from build123d import *

# Parameters (mm, degrees)
SKETCH_R     = 2.2
PAD_DEPTH    = 4
PAD001_DEPTH = 11
POCKET_DEPTH = 2
FILLET_R     = 6.46
CHAMFER_SIZE = 0.6
PAD002_DEPTH = 0.9


with BuildPart() as revolution:
    # Sketch002 → Revolution (revolve)
    with BuildSketch(Plane.XZ):
        Polygon((9.9, 11.25), (10.5, 11.85), (10.5, 7.15), (9.9, 7.75), align=None)
    revolve(axis=Axis((0, 0, 0), (0, 0, 1)))


with BuildPart() as pad002:
    # Sketch → Pad (new body)
    with BuildSketch(Plane.XY):
        with BuildLine():
            Line((-10.212408, -2.440639), (-19.784288, -2.440639))
            Line((-19.784288, -2.440639), (-19.784288, 10.5))
            Line((19.784288, 10.5), (-19.784288, 10.5))
            Line((19.784288, -2.440639), (19.784288, 10.5))
            Line((10.212408, -2.440639), (19.784288, -2.440639))
            ThreePointArc((7.424621, -7.424621), (9.163854, -5.125795), (10.212408, -2.440639))
            Line((5.674532, -5.674532), (7.424621, -7.424621))
            ThreePointArc((5.674532, -5.674532), (0, 8.025), (-5.674532, -5.674532))
            Line((-5.674532, -5.674532), (-7.424621, -7.424621))
            ThreePointArc((-10.212408, -2.440639), (-9.163854, -5.125795), (-7.424621, -7.424621))
        make_face()
        with Locations((13.859288, 4.029681)):
            Circle(SKETCH_R, mode=Mode.SUBTRACT)
        with Locations((-13.859288, 4.029681)):
            Circle(SKETCH_R, mode=Mode.SUBTRACT)
    extrude(amount=PAD_DEPTH)

    # Sketch001 → Pad001 (new body)
    with BuildSketch(Plane.XY.offset(4)):
        with BuildLine():
            ThreePointArc((5.674532, -5.674532), (0, 8.025), (-5.674532, -5.674532))
            Line((-5.674532, -5.674532), (-7.424621, -7.424621))
            ThreePointArc((7.424621, -7.424621), (0, 10.5), (-7.424621, -7.424621))
            Line((5.674532, -5.674532), (7.424621, -7.424621))
        make_face()
    extrude(amount=PAD001_DEPTH)

    # Cut: cut Revolution
    add(revolution.part, mode=Mode.SUBTRACT)

    # Sketch003 → Pocket (cut)
    with BuildSketch(Plane.XY.offset(4)):
        Polygon((17.812321, 3.059611), (16.675909, 6.968072), (12.722877, 7.938142), (9.906256, 4.99975), (11.042667, 1.091289), (14.995699, 0.121219), align=None)
        Polygon((-17.812321, 3.059611), (-14.995699, 0.121219), (-11.042667, 1.091289), (-9.906256, 4.99975), (-12.722877, 7.938142), (-16.675909, 6.968072), align=None)
    extrude(amount=-POCKET_DEPTH, mode=Mode.SUBTRACT)

    # Fillet
    fillet_edges = [pad002.edges().sort_by_distance(p)[0] for p in [
        (19.784288, -2.440639, 2),
        (19.784288, 10.5, 2),
        (-19.784288, 10.5, 2),
        (-19.784288, -2.440639, 2),
    ]]
    fillet(fillet_edges, radius=FILLET_R)

    # Chamfer
    chamfer_edges = [pad002.edges().sort_by_distance(p)[0] for p in [
        (0, 10.5, 0),
        (17.892198, 8.60791, 0),
        (-17.892198, 8.60791, 0),
    ]]
    chamfer(chamfer_edges, length=CHAMFER_SIZE)

    # Sketch004 → Pad002 (new body)
    with BuildSketch(Plane(origin=(0, 0, 0), x_dir=(1, 0, 0), z_dir=(0, 0, -1))):
        with BuildLine():
            ThreePointArc((-4.949747, 4.949747), (0, -7), (4.949747, 4.949747))
            Line((4.949747, 4.949747), (5.674532, 5.674532))
            ThreePointArc((-5.674532, 5.674532), (0, -8.025), (5.674532, 5.674532))
            Line((-5.674532, 5.674532), (-4.949747, 4.949747))
        make_face()
    extrude(amount=-PAD002_DEPTH)


solid = pad002.part
Geometry check sheet. Reference: the model listing, model coordinates, mm. A direction names the side the tool comes from. Give positions to 0.01 mm unless a question says otherwise; leave off trailing zeros. Loops run counter-clockwise (first coordinate to the right, second up) from the corner with the lowest first, then second, coordinate; pieces in that order, holes last. Notation, with made-up numbers: M 82,64.25 L 92,64.25 A30 cw 92,87.25 Z; hole C -13.75,-27 d7. An arc over 180 degrees is marked long. Answer as a JSON object with one key per item and string values. Group by question number.
Item 1: Mould release check, pull along Y, two halves, no side actions. Record for faces 1 (the flat face through (0, 9, 0)), 2 (the flat face through (0, 10.5, 2)), 3 (the flat face through (10.467, 3.073, 3.014)): pulls with the +Y half, pulls with the -Y half, needs draft (parallel to the pull), parting line crosses it, or undercut.
Item 2: Gauge pin test, flat ends, axial feed: pin 1 (2 mm diameter, centred on x = 5, z = 8.5, fed in from +Y); pin 2 (8.5 mm diameter, centred on x = 0, y = 0, fed in from +Z); pin 3 (2 mm diameter, centred on y = 7.5, z = 7.5, fed in from -X); pin 4 (2 mm diameter, centred on x = 2.5, z = 3, fed in from -Y). Record the tip position at first contact, or that the pin passes through.
Item 3: Material ranges on L1, parallel to Z at x = 12.5, y = 0.25; L2, parallel to X at y = 6.5, z = 12; L3, parallel to X at y = -3.75, z = 2, recorded low to high.
Item 4: Sectioned sample at C-C on z = 4.75. Record the boundary of the cut face in (x, y) (3 decimals).
Item 5: Sectioned sample at A-A on z = 2.5. Record the boundary of the cut face in (x, y) (3 decimals).
Item 6: Access from +Z, -Z, +X, -X, +Y, -Y to the whole of each face (thin tool, end or side, straight path). Record for faces 4 (the conical face through (0.332, 10.057, 7.588)), 5 (the flat face through (-11.295, 6.448, 3.014)), 6 (the flat face through (-12, -2.441, 2)).
Item 7: Sectioned sample at B-B on z = 8.5. Record the boundary of the cut face in (x, y) (3 decimals), plus the area to 3 significant figures.
Findings below:
{
 "1": {"face 1": "needs draft", "face 2": "pulls with the +Y half", "face 3": "undercut"},
 "2": {"pin 1": "y = 9.06", "pin 2": "through", "pin 3": "x = -8.2", "pin 4": "y = 7.22"},
 "3": {"L1": "0 to 4", "L2": "-8.25 to -4.71, 4.71 to 8.25", "L3": "-9.81 to -7.09, 7.09 to 9.81"},
 "4": {"outline": "M -7.425,-7.425 L -5.675,-5.675 A8.025 cw long 5.675,-5.675 L 7.425,-7.425 A10.5 ccw long Z"},
 "5": {"outline": "M -19.784,4.019 A6.46 ccw -13.324,-2.441 L -10.212,-2.441 A10.5 ccw -7.425,-7.425 L -5.675,-5.675 A8.025 cw long 5.675,-5.675 L 7.425,-7.425 A10.5 ccw 10.212,-2.441 L 13.324,-2.441 A6.46 ccw 19.784,4.019 L 19.784,4.04 A6.46 ccw 13.324,10.5 L -13.324,10.5 A6.46 ccw -19.784,4.04 Z; hole M -17.812,3.06 L -14.996,0.121 L -11.043,1.091 L -9.906,5 L -12.723,7.938 L -16.676,6.968 Z; hole M 9.906,5 L 11.043,1.091 L 14.996,0.121 L 17.812,3.06 L 16.676,6.968 L 12.723,7.938 Z"},
 "6": {"face 4": "none", "face 5": "+Z", "face 6": "+Z, -Z, -X, -Y"},
 "7": {"outline": "M -7,-7 L -5.675,-5.675 A8.025 cw long 5.675,-5.675 L 7,-7 A9.9 ccw long Z", "area": "79.2 mm2"}
}
